Print and shaded views of the part. All mm, measured from the part's lowest x, y and z. A direction names the side the tool comes from. Round coordinates to 2 decimals unless told otherwise and drop trailing zeros. Loops run counter-clockwise (first coordinate to the right, second up) from the corner with the lowest first, then second, coordinate; pieces in that order, holes last. Notation, with made-up numbers: (0, 48) -> (58, 48) arc R35 ccw to (58, 81) -> close; hole circle Ø7 at (60, -34.75). An arc over 180 degrees is marked (long way). Answer as CSV lines item,"result".
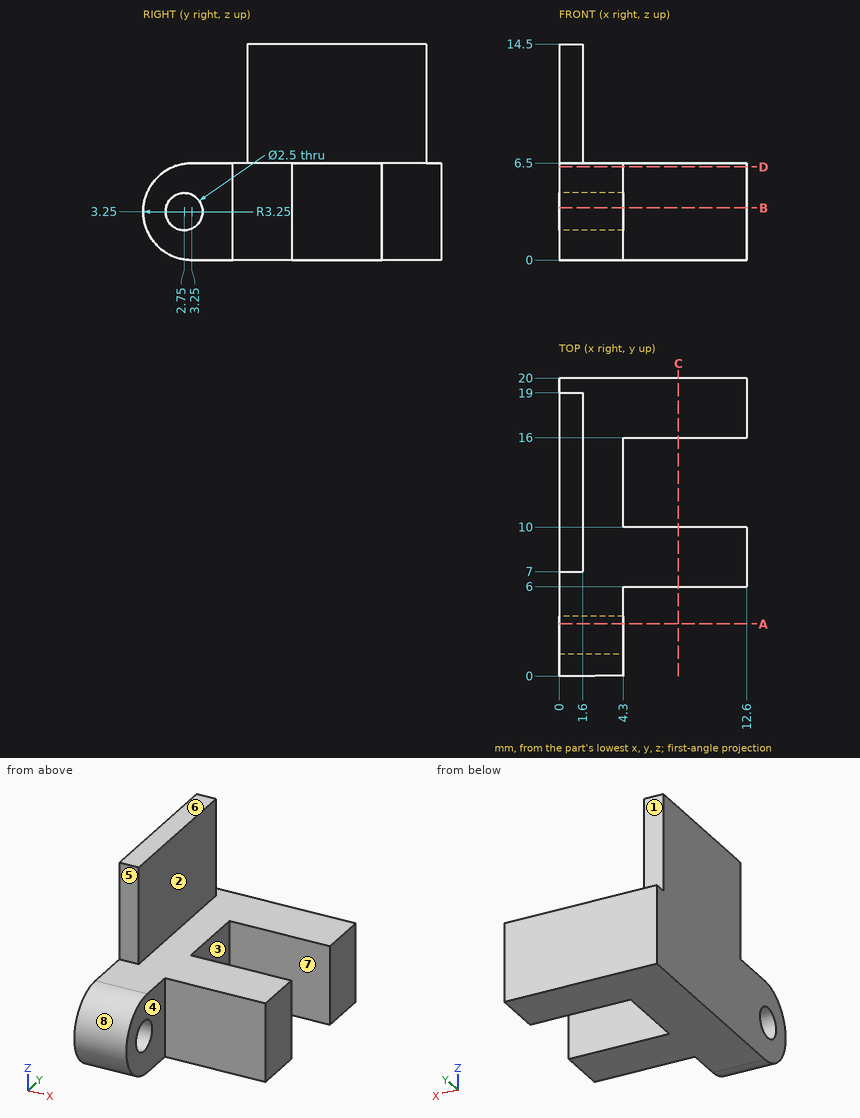
Q1. Saw through at B-B, the plane z = 3.5. Write the cut outline in (x, y).
Geometry results:
outline,"(0, 0.01) -> (4.3, 0.01) -> (4.3, 1.53) -> (0, 1.53) -> close; (0, 3.97) -> (4.3, 3.97) -> (4.3, 6) -> (12.6, 6) -> (12.6, 10) -> (4.3, 10) -> (4.3, 16) -> (12.6, 16) -> (12.6, 20) -> (0, 20) -> close"
Q2. Saw through at A-A, the plane y = 3.5. Write the cut outline in (x, z).
Geometry results:
outline,"(0, 0) -> (4.3, 0) -> (4.3, 2.25) -> (0, 2.25) -> close; (0, 4.25) -> (4.3, 4.25) -> (4.3, 6.5) -> (0, 6.5) -> close"
Q3. Which spindle directions (+Z, -Z, +X, -X, +Y, -Y) get a long thin tool onto all of the face, cutting with end or side? Do the marked faces 1, 2, 3, 4 and 5. Say none if no direction does.
Geometry results:
face 1,"+Z, +X, -X, +Y"
face 2,"+Z, +X, +Y, -Y"
face 3,"+Z, -Z, +X"
face 4,"+Z, -Z, +X, -Y"
face 5,"+Z, +X, -X, -Y"
Q4. Saw through at D-D, the plane z = 6.25. Write the cut outline in (x, y).
Geometry results:
outline,"(0, 2) -> (4.3, 2) -> (4.3, 6) -> (12.6, 6) -> (12.6, 10) -> (4.3, 10) -> (4.3, 16) -> (12.6, 16) -> (12.6, 20) -> (0, 20) -> close"
Q5. Two-plate mould, pull along Y, no slides. Class the marked faces 6, 7 and 8: pulls with the +Y half, pulls with the -Y half, needs draft (parallel to the pull), parting line crosses it, or undercut.
Geometry results:
face 6,"needs draft"
face 7,"undercut"
face 8,"pulls with the -Y half"
Q6. Drill centre lines: line 1 along Y through (x, z) = (11, 4.5); line 2 along X through (y, z) = (13, 9.75); line 3 along Z through (x, y) = (11.75, 8.75). Where is each one in solid material? Low to high.
Geometry results:
line 1,"6 to 10, 16 to 20"
line 2,"0 to 1.6"
line 3,"0 to 6.5"
Q7. Saw through at C-C, the plane x = 8. Write the cut outline in (y, z).
Geometry results:
outline,"(6, 0) -> (10, 0) -> (10, 6.5) -> (6, 6.5) -> close; (16, 0) -> (20, 0) -> (20, 6.5) -> (16, 6.5) -> close"
Q8. Drop flat-ended pins along their axis: P1, Ø1, axis at y = 16, z = 10.5, coming from the +X side; P2, Ø1, axis at x = 10.5, z = 5, coming from the -Y side; P3, Ø5, axis at y = 12, z = 3, coming from the +X side; P4, Ø4, axis at x = 6.5, y = 9, coming from the +Z side. Give the stop position or say it passes through.
Geometry results:
P1,"x = 1.6"
P2,"y = 6"
P3,"x = 12.6"
P4,"z = 6.5"
